Read the model definition and answer for the solid it produces. Units are mm, in the model's axes. A direction names the side the tool comes from. Round coordinates to 2 decimals unless told otherwise and drop trailing zeros. Order: outer loops, then holes, each group sorted by start corner. A loop starts at its lowest first (then second) coordinate and runs counter-clockwise, first axis right, second up. Notation, with made-up numbers: (-31.5, 75.5) - (5.5, 75.5) arc R20 cw to (5.5, 112.5) - close; hole circle Ø6 at (-29.75, -36). An arc over 180 degrees is marked (long way). Answer as a JSON object with one key per item and string values. Group by question number.
Q1. A cutting plane is placed at C-C on y = 35. Determine the outline of the cut face in (x, z), and give its area (3 significant figures).
Q2. Consider line 1 (Y direction, x = 0, z = -2); line 2 (Y direction, x = 0, z = -7.75); line 3 (X direction, y = 9, z = -4). Determine where each line is inside the solid, lowest interval first.
Q3. The mould has two halves that part along Y. Classify faces 3 (the flat face through (44.551, 8.593, -3.895)), 4 (the flat face through (7.327, 25.69, -3.895)), 5 (the flat face through (13, 19, -4)), 6 (the cylindrical face through (22.36, 3.94, -4.31)): pulls with the +Y half, pulls with the -Y half, needs draft (parallel to the pull), parting line crosses it, or undercut.
Q4. A tool of negligible diameter and unlimited length cuts with its end or side. For faces 1 (the cylindrical face through (-14.515, 17.341, -4.31)), 2 (the flat face through (0, 38.5, -4)), from which of +Z, -Z, +X, -X, +Y, -Y can it reach the whole face along a straight path? Write none if from no direction.
Q5. A cutting plane is placed at A-A on y = 0. Determine the outline of the cut face in (x, z).
Q6. A cutting plane is placed at B-B on x = 37.5. Determine the outline of the cut face in (y, z), and give its area (3 significant figures).
Q7. Given pin 1 Ø3.5 at (y, z) = (11, -5) entering from -X; pin 2 Ø5 at (x, y) = (-26, -11) entering from +Z; pin 3 Ø8.5 at (x, y) = (0, 0) entering from -Z; pin 4 Ø2.5 at (x, z) = (-24.5, -2.5) entering from -Y, each flat-ended and moving along its own axis, determine where each tip first touches the part or whether it passes through.
Q8. A cutting plane is placed at D-D on z = -4.5. Count the separate pieces of the cut face and the enclosed holes in it, and give its area (3 significant figures).
```python
from build123d import *

# Parameters (mm, degrees)
F0_R     = 11.1
F0_R_2   = 7
F1_DEPTH = 8.5
F2_DEPTH = 7.9
F3_DEPTH = 7.2
F4_COUNT = 3
F5_R     = 3.6339158304


# Not quite as in the source:
# - a feature names something its author has since deleted; it is built from what else it names


with BuildPart() as f1:
    # F0 (on Top) → F1 (new body)
    with BuildSketch(Plane.XY):
        with BuildLine():
            ThreePointArc((-11.1881680787, 23.3799626101), (3.4317499164, 17.4611367137), (13, 30))
            ThreePointArc((13, 30), (3.4317499164, 42.5388632863), (-11.1881680787, 36.6200373899))
            ThreePointArc((-11.1881680787, 36.6200373899), (-35.2898051844, 31.4974370391), (-13, 20.9953167593))
            ThreePointArc((-13, 20.9953167593), (-12.0251844061, 22.1352903789), (-11.1881680787, 23.3799626101))
        make_face()
        Polygon((-17.4962580338, 38.5157601447), (-12.5614324777, 30.0316084449), (-17.4415106013, 21.5158483002), (-27.2564142809, 21.4842398553), (-32.1912398369, 29.9683915551), (-27.3111617133, 38.4841516998), align=None, mode=Mode.SUBTRACT)
        Polygon((4.9074772881, 38.5), (9.8149545762, 30), (4.9074772881, 21.5), (-4.9074772881, 21.5), (-9.8149545762, 30), (-4.9074772881, 38.5), align=None, mode=Mode.SUBTRACT)
        with BuildLine():
            ThreePointArc((-13, 0), (0, -13), (13, 0))
            ThreePointArc((13, 0), (0, 13), (-13, 0))
        make_face()
        Circle(F0_R, mode=Mode.SUBTRACT)
        Circle(F0_R)
        Circle(F0_R_2, mode=Mode.SUBTRACT)
        Polygon((4.9074772881, 21.5), (9.8149545762, 30), (4.9074772881, 38.5), (-4.9074772881, 38.5), (-9.8149545762, 30), (-4.9074772881, 21.5), align=None)
        Polygon((-17.4415106013, 21.5158483002), (-12.5614324777, 30.0316084449), (-17.4962580338, 38.5157601447), (-27.3111617133, 38.4841516998), (-32.1912398369, 29.9683915551), (-27.2564142809, 21.4842398553), align=None)
        with BuildLine():
            ThreePointArc((-13, 0), (0, 13), (13, 0))
            Line((13, 0), (13, 30))
            ThreePointArc((13, 30), (3.4317499164, 17.4611367137), (-11.1881680787, 23.3799626101))
            ThreePointArc((-11.1881680787, 23.3799626101), (-12.0251844061, 22.1352903789), (-13, 20.9953167593))
            Line((-13, 20.9953167593), (-13, 0))
        make_face()
    extrude(amount=-F1_DEPTH)

    # F0 (on Top) → F2 (cut)
    with BuildSketch(Plane.XY):
        Polygon((4.9074772881, 21.5), (9.8149545762, 30), (4.9074772881, 38.5), (-4.9074772881, 38.5), (-9.8149545762, 30), (-4.9074772881, 21.5), align=None)
        Polygon((-17.4415106013, 21.5158483002), (-12.5614324777, 30.0316084449), (-17.4962580338, 38.5157601447), (-27.3111617133, 38.4841516998), (-32.1912398369, 29.9683915551), (-27.2564142809, 21.4842398553), align=None)
    extrude(amount=-F2_DEPTH, mode=Mode.SUBTRACT)

    # F0 (on Top) → F3 (cut)
    with BuildSketch(Plane.XY):
        Circle(F0_R)
        Circle(F0_R_2, mode=Mode.SUBTRACT)
    extrude(amount=-F3_DEPTH, mode=Mode.SUBTRACT)

    # F4: F1 ×3 about axis
    f4_axis = Axis((0, 0, 0), (0, 0, 1))


with BuildPart() as f1_1:
    add(f1.part)
    for i in range(1, F4_COUNT):
        add(f1.part.rotate(f4_axis, i * 360 / F4_COUNT))

    # F5
    f5_edges = [f1_1.edges().sort_by_distance(p)[0] for p in [
        (-13, 20.995317, -4.25),
        (-11.188168, 36.620037, -4.25),
        (-11.682478, -21.755989, -4.25),
        (-26.119799, -27.999256, -4.25),
        (37.307967, -8.620781, -4.25),
        (24.682478, 0.760672, -4.25),
    ]]
    fillet(f5_edges, radius=F5_R)


solid = f1_1.part
```
Result set:
{
 "1": {"outline": "(-34.38, -8.5) - (12, -8.5) - (12, 0) - (6.93, 0) - (6.93, -7.9) - (-6.93, -7.9) - (-6.93, 0) - (-15.45, 0) - (-15.45, -7.9) - (-29.31, -7.9) - (-29.31, 0) - (-34.38, 0) - close", "area": "175 mm²"},
 "2": {"line 1": "y = -15.01 to -11.1, 11.1 to 21.5, 38.5 to 43", "line 2": "y = -15.01 to -7, 7 to 21.5, 38.5 to 43", "line 3": "x = -13 to -6.5, 6.5 to 13, 25.02 to 30.02, 44.31 to 49.32"},
 "3": {"face 3": "undercut", "face 4": "undercut", "face 5": "needs draft", "face 6": "pulls with the +Y half"},
 "4": {"face 1": "+Z, -Z", "face 2": "+Z"},
 "5": {"outline": "(-26, -8.5) - (-7, -8.5) - (-7, -7.2) - (-11.1, -7.2) - (-11.1, 0) - (-26, 0) - close; (7, -8.5) - (49.41, -8.5) - (49.41, 0) - (44.46, 0) - (44.46, -7.9) - (29.88, -7.9) - (29.88, 0) - (11.1, 0) - (11.1, -7.2) - (7, -7.2) - close"},
 "6": {"outline": "(-21.03, -8.5) - (17.37, -8.5) - (17.37, 0) - (12.88, 0) - (12.88, -7.9) - (-4.12, -7.9) - (-4.12, 0) - (-21.03, 0) - close", "area": "192 mm²"},
 "7": {"pin 1": "stops at x = -13", "pin 2": "stops at z = -7.9", "pin 3": "passes through", "pin 4": "stops at y = -44.25"},
 "8": {"separate pieces": "1", "enclosed holes": "7", "area": "2,470 mm²"}
}
